from build123d import *

# Parameters (mm, degrees)
BOSS_EXTRUDE1_DEPTH = 3.175
FILLET1_START       = -4
FILLET1_DEPTH       = 8
SKETCH2_W           = 12.7
SKETCH2_H           = 6.35
BOSS_EXTRUDE2_DEPTH = 6.35


with BuildPart() as part:
    # Sketch1 → Boss-Extrude1 (new, symmetric)
    with BuildSketch(Plane(origin=(0, 0, 0), x_dir=(1, 0, 0), z_dir=(0, 1, 0))):
        with BuildLine():
            Line((-54.202443258, -43.180856192), (-66.902443258, -43.180856192))
            ThreePointArc((-66.902443258, -43.180856192), (-33.83954697, -60.596845897), (-3.959326756, -38.154826194))
            ThreePointArc((-3.959326756, -38.154826194), (-12.780230261, -45.982812034), (-24.23600367, -43.180856192))
            Line((-24.23600367, -43.180856192), (-41.502443258, -43.180856192))
            Line((-41.502443258, -43.180856192), (-54.202443258, -43.180856192))
        make_face()
    extrude(amount=BOSS_EXTRUDE1_DEPTH, both=True)

    # Fillet1: read off the stored shape, not the designer's step
    # Fillet1 outline → Fillet1 (cut)
    with BuildSketch(Plane(origin=(0, 0, 0), x_dir=(1, 0, 0), z_dir=(0, 1, 0)).offset(FILLET1_START)):
        with BuildLine():
            ThreePointArc((-11.522510786, -45.600981794), (-9.683883576, -46.182242141), (-9.76258933, -48.108954111))
            ThreePointArc((-9.76258933, -48.108954111), (-6.447625568, -43.372863288), (-3.959326789, -38.15482628))
            ThreePointArc((-3.959326789, -38.15482628), (-6.925777422, -42.705856679), (-11.522510786, -45.600981794))
        make_face()
    extrude(amount=FILLET1_DEPTH, mode=Mode.SUBTRACT)

    # Sketch2 → Boss-Extrude2 (add)
    with BuildSketch(Plane(origin=(0, 3.175, 0), x_dir=(1, 0, 0), z_dir=(0, 1, 0))):
        with Locations((-45.569223464, -40.005856192)):
            Rectangle(SKETCH2_W, SKETCH2_H)
    extrude(amount=-BOSS_EXTRUDE2_DEPTH)


solid = part.part
Source: CAD feature listing. Evaluate the final solid. Frame: model axes, mm. A direction names the side the tool comes from. Coordinates: 2 decimals unless noted, no trailing zeros. Loops run counter-clockwise (first coordinate to the right, second up) from the corner with the lowest first, then second, coordinate; pieces in that order, holes last. Notation, with made-up numbers: (37.25, -24.75) - (54.25, -24.75) arc R12 ccw to (54.25, -15.75) - close; hole circle Ø3 at (67.5, 14). An arc over 180 degrees is marked (long way). One line per question, with ' | ' between items.
1) Pull-direction query (X, two-part tool) for faces 1 (the face through (-39, 3.175, 49)), 2 (the face through (-40.089, 0.044, 60.535)), 3 (the face through (-18.12, 0.04, 46.15)); classes: released by +X, released by -X, zero draft, split by the parting line, or undercut.
Report:
face 1: zero draft | face 2: split by the parting line | face 3: undercut
2) Section C-C, the plane x = -53.5. Return loops of the section in (y, z) (3 decimals).
Report:
outline: (-3.175, 43.181) - (3.175, 43.181) - (3.175, 56.357) - (-3.175, 56.357) - close
3) Set-up query: faces 4 (the face through (-46, 0, 36.831)), 5 (the face through (-59, 0, 43.181)), 6 (the face through (-39.219, 0, 40)). Return all of +Z, -Z, +X, -X, +Y, -Y with unobstructed straight access to the full face (end or side cutting, diameter ignored); none if empty.
Report:
face 4: -Z, +X, -X, +Y, -Y | face 5: -Z, -X, +Y, -Y | face 6: -Z, +X, +Y, -Y
4) First-contact query: P1, Ø3, axis at y = 0.5, z = 49.5, coming from the +X side; P2, Ø2, axis at y = 1, z = 51, coming from the -X side; P3, Ø1.5, axis at y = 1, z = 49.5, coming from the -X side. Flat tips, straight axial feed; report the tip coordinate or a pass-through.
Report:
P1: stops at x = -9.68 | P2: stops at x = -61.78 | P3: stops at x = -62.93
5) Section B-B, the plane z = 42. Return loops of the section in (x, y) (3 decimals).
Report:
outline: (-51.919, -3.175) - (-39.219, -3.175) - (-39.219, 3.175) - (-51.919, 3.175) - close
6) Line query: line 1 along X through (y, z) = (0.5, 42.5); line 2 along Z through (x, y) = (-31, -2.25); line 3 along Z through (x, y) = (-49, 0.25). Output: solid intervals per line, ascending.
Report:
line 1: x = -51.92 to -39.22 | line 2: z = 43.18 to 60.25 | line 3: z = 36.83 to 58.44
